Check sheet for the modelled part. Datum: model origin and axes. Units: mm. A direction names the side the tool comes from. Round coordinates to 2 decimals unless told otherwise and drop trailing zeros. Order: outer loops, then holes, each group sorted by start corner. A loop starts at its lowest first (then second) coordinate and runs counter-clockwise, first axis right, second up.
Autodesk Inventor part; units mm, degrees
ref_plane "YZ Plane" through (0, 0, 0) normal (1, 0, 0) x (0, 1, 0)
ref_plane "XZ Plane" through (0, 0, 0) normal (0, 1, 0) x (-1, 0, 0)
ref_plane "XY Plane" through (0, 0, 0) normal (0, 0, 1) x (1, 0, 0)
sketch "Sketch1" plane through (0, 0, 0) normal (0, 1, 0) x (-1, 0, 0)
  line L0 (-50.8, 50.8) -> (50.8, 50.8)
  line L1 (50.8, 50.8) -> (50.8, -50.8)
  line L2 (50.8, -50.8) -> (-50.8, -50.8)
  line L3 (-50.8, -50.8) -> (-50.8, 50.8)
  line L4 (-63.5, 63.5) -> (63.5, 63.5)
  line L5 (63.5, 63.5) -> (63.5, -63.5)
  line L6 (63.5, -63.5) -> (-63.5, -63.5)
  line L7 (-63.5, -63.5) -> (-63.5, 63.5)
  point P0 (0, 0)
  dimension "d0" = 101.6
  dimension "d1" = 101.6
  dimension "d2" = 127
  dimension "d3" = 127
  dimension "d4" = 63.5
  dimension "d5" = 63.5
  dimension "d6" = 50.8
  dimension "d7" = 50.8
extrude "Extrusion1" add sketch "Sketch1" against normal blind 38.1
fillet "Fillet1" radius 12.7 4 edges at (-50.8, -19.05, -50.8) (50.8, -19.05, -50.8) (-50.8, -19.05, 50.8) (50.8, -19.05, 50.8)
sketch "Sketch3" plane through (0, 0, 0) normal (0, 1, 0) x (1, 0, 0)
  line L0 (-63.5, 63.5) -> (63.5, 63.5)
  line L1 (63.5, 63.5) -> (63.5, -63.5)
  line L2 (63.5, -63.5) -> (-63.5, -63.5)
  line L3 (-63.5, -63.5) -> (-63.5, 63.5)
  point P0 (0, 0)
extrude "Extrusion2" add sketch "Sketch3" along normal blind 12.7
sketch "Sketch4" plane through (0, 12.7, 0) normal (0, 1, 0) x (1, 0, 0)
  line L0 (63.5, -63.5) -> (63.5, 63.5)
  line L1 (63.5, 63.5) -> (-63.5, 63.5)
  circle A0 centre (38.1, 38.1) radius 3.175
  circle A1 centre (-69.85, 38.1) radius 3.175
  circle A2 centre (38.1, -69.85) radius 3.175
  circle A3 centre (-69.85, -69.85) radius 3.175
  point P0 (0, 0)
  dimension "d13" = 6.35
  dimension "d14" = 25.4
  dimension "d15" = 25.4
  dimension "d18" = 107.95
  dimension "d21" = 107.95
extrude "Extrusion3" cut sketch "Sketch4" against normal up to next
sketch "Sketch5" plane through (0, 12.7, 0) normal (0, 1, 0) x (1, 0, 0)
  circle A0 centre (50.8, -57.15) radius 3.175
  circle A1 centre (38.1, 38.1) radius 3.175
  circle A2 centre (-57.15, 50.8) radius 3.175
  circle A3 centre (-57.15, -57.15) radius 3.175
  circle A4 centre (-57.15, -57.15) radius 6.35
  circle A5 centre (-57.15, 50.8) radius 6.35
  circle A6 centre (38.1, 38.1) radius 6.35
  circle A7 centre (50.8, -57.15) radius 6.35
  point P0 (0, 0)
  dimension "d26" = 12.7
  dimension "d27" = 12.7
  dimension "d28" = 12.7
  dimension "d29" = 12.7
extrude "Extrusion4" [suppressed]
sketch "Sketch6" plane through (0, 12.7, 0) normal (0, 1, 0) x (1, 0, 0)
  line L0 (-45.1827, 25.9215) -> (43.7173, 25.9215)
  line L1 (43.7173, 25.9215) -> (43.7173, -43.9285)
  line L2 (43.7173, -43.9285) -> (-45.1827, -43.9285)
  line L3 (-45.1827, -43.9285) -> (-45.1827, 25.9215)
  line L4 (-51.5327, 32.2715) -> (50.0673, 32.2715)
  line L5 (50.0673, 32.2715) -> (50.0673, -50.2785)
  line L6 (50.0673, -50.2785) -> (-51.5327, -50.2785)
  line L7 (-51.5327, -50.2785) -> (-51.5327, 32.2715)
  point P0 (0, 0)
  dimension "d32" = 69.85
  dimension "d33" = 88.9
  dimension "d36" = 6.35
  dimension "d37" = 6.35
  dimension "d38" = 6.35
  dimension "d39" = 6.35
extrude "Extrusion5" add sketch "Sketch6" along normal blind 25.4
sketch "Sketch7" plane through (0, 12.7, 0) normal (0, 1, 0) x (1, 0, 0)
  line L0 (43.7173, -43.9285) -> (43.7173, 25.9215)
  line L1 (43.7173, 25.9215) -> (-45.1827, 25.9215)
  line L2 (-45.1827, 25.9215) -> (43.7173, 25.9215)
  line L3 (43.7173, 25.9215) -> (43.7173, -43.9285)
  line L4 (43.7173, -43.9285) -> (-45.1827, -43.9285)
  line L5 (-45.1827, -43.9285) -> (-45.1827, 25.9215)
  point P0 (0, 0)
  point P1 (63.5839, -35.7281)
  point P2 (63.5, 18.4248)
extrude "Extrusion6" cut sketch "Sketch7" against normal up to next
properties part number "Case1"
Item 1: Scan lines: line 1 along Z through (x, y) = (38.1, 3.25) (1 decimal); line 2 along X through (y, z) = (2.5, -38.1) (3 decimals); line 3 along X through (y, z) = (3.5, 43.5). Record each from-to range of solid material in increasing order.
Answer:
line 1: z = -63.5 to -41.3, -34.9 to -25.9, 43.9 to 63.5
line 2: x = -63.5 to 34.925, 41.275 to 63.5
line 3: x = -63.5 to -45.18, 43.72 to 63.5
Item 2: Sectioned sample at C-C (z = -30). Record the cut outline in (x, y).
Answer:
outline: (-63.5, -38.1) - (-50.8, -38.1) - (-50.8, 0) - (50.8, 0) - (50.8, -38.1) - (63.5, -38.1) - (63.5, 12.7) - (50.07, 12.7) - (50.07, 38.1) - (-51.53, 38.1) - (-51.53, 12.7) - (-63.5, 12.7) - close
Item 3: Sectioned sample at D-D (y = -26.5). Record the cut outline in (x, z), and give its area (3 significant figures).
Answer:
outline: (-63.5, -63.5) - (63.5, -63.5) - (63.5, 63.5) - (-63.5, 63.5) - close; hole (-50.8, -38.1) arc R12.7 ccw to (-38.1, -50.8) - (38.1, -50.8) arc R12.7 ccw to (50.8, -38.1) - (50.8, 38.1) arc R12.7 ccw to (38.1, 50.8) - (-38.1, 50.8) arc R12.7 ccw to (-50.8, 38.1) - close
area: 5,940 mm2
Item 4: Release check for a two-part mould opening along X. For faces 1 (the flat face through (43.717, 19, 9)), 2 (the flat face through (-63.5, -13, 1)), 3 (the flat face through (-45.183, 19, 9)), 4 (the flat face through (-1, -13, -63.5)) record: released by +X, released by -X, zero draft, split by the parting line, or undercut.
Answer:
face 1: undercut
face 2: released by -X
face 3: undercut
face 4: zero draft
Item 5: Sectioned sample at A-A (y = 14.5). Record the cut outline in (x, z), and give its area (3 significant figures).
Answer:
outline: (-51.53, -32.27) - (50.07, -32.27) - (50.07, 50.28) - (-51.53, 50.28) - close; hole (-45.18, -25.92) - (43.72, -25.92) - (43.72, 43.93) - (-45.18, 43.93) - close
area: 2,180 mm2
Item 6: Sectioned sample at B-B (x = -1). Record the cut outline in (y, z), and give its area (3 significant figures).
Answer:
outline: (-38.1, -63.5) - (12.7, -63.5) - (12.7, -32.27) - (38.1, -32.27) - (38.1, -25.92) - (0, -25.92) - (0, -50.8) - (-38.1, -50.8) - close; (-38.1, 50.8) - (0, 50.8) - (0, 43.93) - (38.1, 43.93) - (38.1, 50.28) - (12.7, 50.28) - (12.7, 63.5) - (-38.1, 63.5) - close
area: 2,020 mm2
Item 7: Access from +Z, -Z, +X, -X, +Y, -Y to the whole of each face (thin tool, end or side, straight path). Record for faces 5 (the flat face through (63.5, -13, -1)), 6 (the flat face through (0, 25, 50.278)), 7 (the cylindrical face through (-47.18, -19.32, -46.98)), 8 (the flat face through (0, 19, 43.928)), 9 (the flat face through (-1, 25, -32.272)).
Answer:
face 5: +Z, -Z, +X, +Y, -Y
face 6: +Z, +X, -X, +Y
face 7: -Y
face 8: +Y, -Y
face 9: -Z, +X, -X, +Y
Item 8: Go/stop test with flat-tipped pins: P1, Ø7.5, axis at x = 18, y = 29.5, coming from the +Z side; P2, Ø20.5, axis at x = -20, y = 31.5, coming from the -Z side; P3, Ø10, axis at x = 38.1, z = -38.1, coming from the -Y side; P4, Ø11.5, axis at y = 15, z = 26, coming from the +X side. Record where each tip stops, or that it passes through.
Answer:
P1: stops at z = 50.28
P2: stops at z = -32.27
P3: stops at y = 0
P4: stops at x = 63.5
